Check sheet for the modelled part. Datum: model origin and axes. Units: mm. Give positions to 0.01 mm unless a question says otherwise; leave off trailing zeros. Order: outer loops, then holes, each group sorted by start corner. A loop starts at its lowest first (then second) coordinate and runs counter-clockwise, first axis right, second up. Notation, with made-up numbers: M 50.25,62 L 69.25,62 A30 cw 69.25,87 Z; hole C -26.75,16.5 d11. An arc over 180 degrees is marked long. Answer in a Markdown table with one row per item. Add a question column.
from build123d import *

# Parameters (mm, degrees)
F0_R          = 24
F1_DEPTH      = 2.5
F4_W          = 12
F4_H          = 2
F5_DEPTH      = 4
F6_W          = 3
F6_H          = 3
F7_DEPTH      = 2.5
F7_DEPTH_BACK = 25


with BuildPart() as f1:
    # F0 (on Top) → F1 (new body)
    with BuildSketch(Plane.XY):
        Circle(F0_R)
    extrude(amount=F1_DEPTH)

    # F4 (on face) → F5 (join)
    with BuildSketch(Plane.XY.offset(2.5)):
        with Locations((12, -2)):
            Rectangle(F4_W, F4_H)
        with Locations((12, 2)):
            Rectangle(F4_W, F4_H)
        with Locations((-12, -2)):
            Rectangle(F4_W, F4_H)
        with Locations((-12, 2)):
            Rectangle(F4_W, F4_H)
    extrude(amount=F5_DEPTH)

    # F6 (on face) → F7 (cut, two sides)
    with BuildSketch(Plane.XY.offset(2.5)) as f7_sk:
        with Locations((12.5, -11.5)):
            Rectangle(F6_W, F6_H)
        with Locations((12.5, -6.5)):
            Rectangle(F6_W, F6_H)
        with Locations((12.5, -1.5)):
            Rectangle(F6_W, F6_H)
        with Locations((12.5, 3.5)):
            Rectangle(F6_W, F6_H)
        with Locations((12.5, 8.5)):
            Rectangle(F6_W, F6_H)
        with Locations((12.5, 13.5)):
            Rectangle(F6_W, F6_H)
        with Locations((7.5, -11.5)):
            Rectangle(F6_W, F6_H)
        with Locations((7.5, -6.5)):
            Rectangle(F6_W, F6_H)
        with Locations((7.5, -1.5)):
            Rectangle(F6_W, F6_H)
        with Locations((7.5, 3.5)):
            Rectangle(F6_W, F6_H)
        with Locations((7.5, 8.5)):
            Rectangle(F6_W, F6_H)
        with Locations((7.5, 13.5)):
            Rectangle(F6_W, F6_H)
        with Locations((2.5, -11.5)):
            Rectangle(F6_W, F6_H)
        with Locations((2.5, -6.5)):
            Rectangle(F6_W, F6_H)
        with Locations((2.5, -1.5)):
            Rectangle(F6_W, F6_H)
        with Locations((2.5, 3.5)):
            Rectangle(F6_W, F6_H)
        with Locations((2.5, 8.5)):
            Rectangle(F6_W, F6_H)
        with Locations((2.5, 13.5)):
            Rectangle(F6_W, F6_H)
        with Locations((-2.5, -11.5)):
            Rectangle(F6_W, F6_H)
        with Locations((-2.5, -6.5)):
            Rectangle(F6_W, F6_H)
        with Locations((-2.5, -1.5)):
            Rectangle(F6_W, F6_H)
        with Locations((-2.5, 3.5)):
            Rectangle(F6_W, F6_H)
        with Locations((-2.5, 8.5)):
            Rectangle(F6_W, F6_H)
        with Locations((-2.5, 13.5)):
            Rectangle(F6_W, F6_H)
        with Locations((-7.5, -11.5)):
            Rectangle(F6_W, F6_H)
        with Locations((-7.5, -6.5)):
            Rectangle(F6_W, F6_H)
        with Locations((-7.5, -1.5)):
            Rectangle(F6_W, F6_H)
        with Locations((-7.5, 3.5)):
            Rectangle(F6_W, F6_H)
        with Locations((-7.5, 8.5)):
            Rectangle(F6_W, F6_H)
        with Locations((-7.5, 13.5)):
            Rectangle(F6_W, F6_H)
        with Locations((-12.5, -11.5)):
            Rectangle(F6_W, F6_H)
        with Locations((-12.5, -6.5)):
            Rectangle(F6_W, F6_H)
        with Locations((-12.5, -1.5)):
            Rectangle(F6_W, F6_H)
        with Locations((-12.5, 3.5)):
            Rectangle(F6_W, F6_H)
        with Locations((-12.5, 8.5)):
            Rectangle(F6_W, F6_H)
        with Locations((-12.5, 13.5)):
            Rectangle(F6_W, F6_H)
    extrude(amount=-F7_DEPTH, mode=Mode.SUBTRACT)
    extrude(f7_sk.sketch, amount=F7_DEPTH_BACK, mode=Mode.SUBTRACT)


solid = f1.part
Q1. Thickness scan on probe 1 along X at (y, z) = (-2, 4.25); probe 2 along Y at (x, z) = (14.5, 3.25); probe 3 along Z at (x, y) = (2.5, -4.5). Record the ranges inside material, lowest first.
Q2. Cross-section at B-B (z = 5). State how many separate pieces and enclosed holes the cut face has, and give its area (3 significant figures).
Q3. Draft check along X on faces 1 (the flat face through (6, -7, 1)), 2 (the flat face through (16, -2, 6.5)). Enter one of: pulls with the +X half, pulls with the -X half, needs draft (parallel to the pull), parting line crosses it, or undercut.
Q4. Cross-section at C-C (x = 0). Record the boundary of the cut face in (y, z).
Q5. Cross-section at A-A (y = 13.5). Record the boundary of the cut face in (x, z), and give its area (3 significant figures).
Q6. Go/stop test with flat-tipped pins: pin 1 (3 mm diameter, centred on x = 3, z = 1.5, fed in from -Y); pin 2 (1.2 mm diameter, centred on y = -6.5, z = 1.5, fed in from +X); pin 3 (0.8 mm diameter, centred on x = -12, z = 1.5, fed in from -Y). Record where each tip stops, or that it passes through.
Values follow:
| question | item | result |
|---|---|---|
| 1 | probe 1 | -18 to -14, -11 to -9, 9 to 11, 14 to 18 |
| 1 | probe 2 | -3 to -1, 1 to 3 |
| 1 | probe 3 | 0 to 2.5 |
| 2 | separate pieces | 6 |
| 2 | enclosed holes | 0 |
| 2 | area | 60.0 mm² |
| 3 | face 1 | undercut |
| 3 | face 2 | needs draft |
| 4 | outline | M -24,0 L 24,0 L 24,2.5 L -24,2.5 Z |
| 5 | outline | M -19.84,0 L -14,0 L -14,2.5 L -19.84,2.5 Z; M -11,0 L -9,0 L -9,2.5 L -11,2.5 Z; M -6,0 L -4,0 L -4,2.5 L -6,2.5 Z; M -1,0 L 1,0 L 1,2.5 L -1,2.5 Z; M 4,0 L 6,0 L 6,2.5 L 4,2.5 Z; M 9,0 L 11,0 L 11,2.5 L 9,2.5 Z; M 14,0 L 19.84,0 L 19.84,2.5 L 14,2.5 Z |
| 5 | area | 54.2 mm² |
| 6 | pin 1 | y = -23.95 |
| 6 | pin 2 | x = 23.26 |
| 6 | pin 3 | y = -21.01 |
